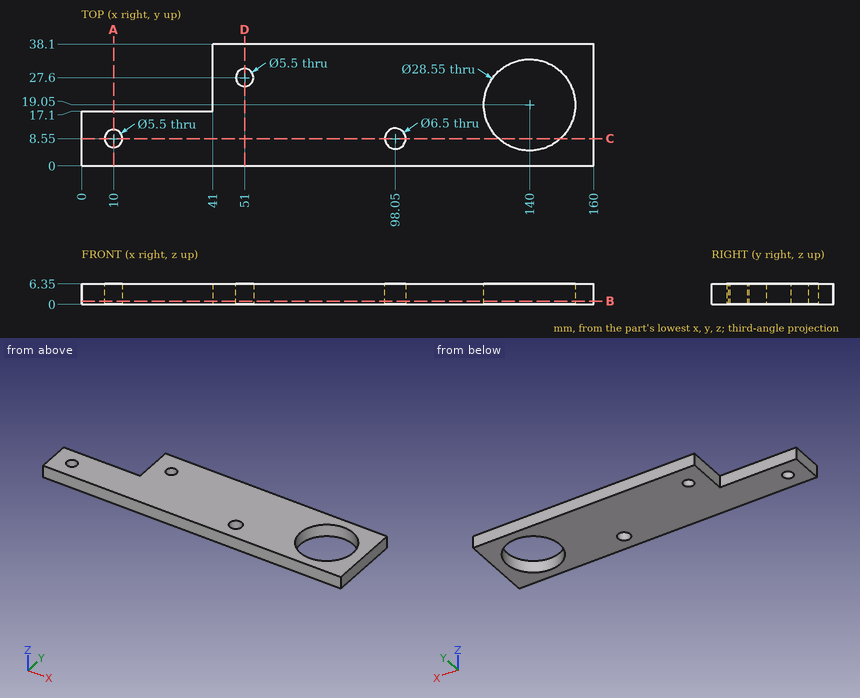
Geometry check sheet. Reference: drawing and pictorial views, mm from the part's lowest x, y, z. Round coordinates to 2 decimals unless told otherwise and drop trailing zeros. Write each loop counter-clockwise with the first axis right and the second up, starting at its lowest first coordinate (ties: lowest second). Pieces come first, ordered by that corner, then holes. Notation, with made-up numbers: (15.25, 39) -> (65.25, 39) arc R32 ccw to (65.25, 72) -> close; hole circle Ø7 at (62.5, 25.25). An arc over 180 degrees is marked (long way). One line per question, with ' | ' between items. Start each with the question number.
1. Sectioned sample at C-C, the plane y = 8.55. Record the cut outline in (x, z), then the cut area to 3 significant figures.
2. Sectioned sample at A-A, the plane x = 10. Record the cut outline in (y, z).
3. Depth check by flat-ended pin: pin 1 (3 mm diameter, centred on y = 26, z = 3.5, fed in from -X). Enter the tip coordinate at first touch or a pass-through.
4. Sectioned sample at B-B, the plane z = 1. Count the separate pieces of the cut face and the enclosed holes in it, then the cut area to 3 significant figures.
5. Sectioned sample at D-D, the plane x = 51. Record the cut outline in (y, z).
6. Scan lines: line 1 along X through (y, z) = (29.5, 5) (1 decimal); line 2 along Y through (x, z) = (140, 4.5) (1 decimal); line 3 along Y through (x, z) = (10, 2). Record each from-to range of solid material in increasing order. Write a range as from..to.
Taken from the geometry:
1) outline: (0, 0) -> (7.25, 0) -> (7.25, 6.35) -> (0, 6.35) -> close; (12.75, 0) -> (94.8, 0) -> (94.8, 6.35) -> (12.75, 6.35) -> close; (101.3, 0) -> (130.33, 0) -> (130.33, 6.35) -> (101.3, 6.35) -> close; (149.67, 0) -> (160, 0) -> (160, 6.35) -> (149.67, 6.35) -> close | area: 817 mm^2
2) outline: (0, 0) -> (5.8, 0) -> (5.8, 6.35) -> (0, 6.35) -> close; (11.3, 0) -> (17.1, 0) -> (17.1, 6.35) -> (11.3, 6.35) -> close
3) pin 1: stops at x = 41
4) separate pieces: 1 | enclosed holes: 4 | area: 4,510 mm^2
5) outline: (0, 0) -> (24.85, 0) -> (24.85, 6.35) -> (0, 6.35) -> close; (30.35, 0) -> (38.1, 0) -> (38.1, 6.35) -> (30.35, 6.35) -> close
6) line 1: x = 41..49, 53..130.3, 149.7..160 | line 2: y = 0..4.8, 33.3..38.1 | line 3: y = 0..5.8, 11.3..17.1
